Geometry: final body of the model. Coordinates: model frame, mm. A direction names the side the tool comes from. Give positions to 0.01 mm unless a question says otherwise; leave off trailing zeros. Loops run counter-clockwise (first coordinate to the right, second up) from the corner with the lowest first, then second, coordinate; pieces in that order, holes last. Notation, with made-up numbers: M 76,-18 L 126,-18 A18 cw 126,11 Z; hole C 83,-23.75 d8. An arc over 180 degrees is marked long. Put each result on its own line as item: value.
```python
from build123d import *

# Parameters (mm, degrees)
SKETCH2_W                = 10
SKETCH2_H                = 7.3
BOSS_EXTRUDE1_DEPTH      = 4.55
SKETCH3_W                = 4.6
SKETCH3_H                = 4.9
CUT_EXTRUDE1_DEPTH       = 3.3
BOSS_EXTRUDE2_DEPTH      = 9.55
BOSS_EXTRUDE2_DEPTH_BACK = 2.7
SKETCH5_W                = 4
SKETCH5_H                = 2
BOSS_EXTRUDE3_REACH      = 19.417
SKETCH13_W               = 5
SKETCH13_H               = 2
SKETCH6_W                = 1.74
SKETCH6_H                = 2
SKETCH6_W_2              = 0.86
SKETCH6_W_3              = 0.8
BOSS_EXTRUDE4_DEPTH      = 0.8
FILLET1_R                = 5
CUT_EXTRUDE2_DEPTH       = 1.2
SKETCH8_R                = 0.65
CUT_EXTRUDE3_DEPTH       = 15.703826033
SKETCH9_R                = 1.125
CUT_EXTRUDE4_DEPTH       = 15.670122699
CUT_EXTRUDE5_REACH       = 20.001
SKETCH10_R               = 0.65
CUT_EXTRUDE6_DEPTH       = 1.3
SKETCH14_W               = 3.4
SKETCH14_H               = 2.947905619
BOSS_EXTRUDE6_DEPTH      = 1.5
SKETCH15_W               = 1.5
SKETCH15_H               = 1.602094381
CUT_EXTRUDE7_DEPTH       = 1.5
FILLET2_R                = 0.25
SKETCH16_W               = 5.8
SKETCH16_H               = 4.9
CUT_EXTRUDE8_DEPTH       = 0.7


with BuildPart() as part:
    # Sketch2 → Boss-Extrude1 (new body)
    with BuildSketch(Plane.XY):
        with Locations((5, 3.65)):
            Rectangle(SKETCH2_W, SKETCH2_H)
    extrude(amount=BOSS_EXTRUDE1_DEPTH)

    # Sketch3 → Cut-Extrude1 (cut)
    with BuildSketch(Plane.XY.offset(4.55)):
        with Locations((4.3, 2.45)):
            Rectangle(SKETCH3_W, SKETCH3_H)
    extrude(amount=-CUT_EXTRUDE1_DEPTH, mode=Mode.SUBTRACT)

    # Sketch5 → Boss-Extrude2 (add, two sides: drawn at the far end of the back side and taken through both)
    with BuildSketch(Plane.XY.offset(-BOSS_EXTRUDE2_DEPTH_BACK)):
        with Locations((-1.4, 4.8)):
            Rectangle(SKETCH5_W, SKETCH5_H)
    extrude(amount=BOSS_EXTRUDE2_DEPTH + BOSS_EXTRUDE2_DEPTH_BACK)

    # Sketch13 → Boss-Extrude3 (add, up to next)
    with BuildSketch(Plane(origin=(0, 0, -2.7), x_dir=(-1, 0, 0), z_dir=(0, 0, -1)), mode=Mode.PRIVATE) as boss_extrude3_sk1:
        with Locations((0.9, 4.8)):
            Rectangle(SKETCH13_W, SKETCH13_H)
    boss_extrude3_tool1 = extrude(boss_extrude3_sk1.sketch, amount=-BOSS_EXTRUDE3_REACH, mode=Mode.PRIVATE) - part.part
    add(boss_extrude3_tool1.solids().sort_by_distance((-0.9, 4.8, -2.7))[0])

    # Sketch6 → Boss-Extrude4 (add)
    with BuildSketch(Plane(origin=(0, 0, -2.7), x_dir=(-1, 0, 0), z_dir=(0, 0, -1))):
        with Locations((0.93, 4.8)):
            Rectangle(SKETCH6_W, SKETCH6_H)
        with Locations((-1.17, 4.8)):
            Rectangle(SKETCH6_W_2, SKETCH6_H)
        with Locations((3, 4.8)):
            Rectangle(SKETCH6_W_3, SKETCH6_H)
    extrude(amount=BOSS_EXTRUDE4_DEPTH)

    # Fillet1
    # the kernel refuses this fillet: 5 mm, written as the material it adds along each edge
    with BuildSketch(Plane(origin=(1.6, 3.8, 0), x_dir=(0, 0, -1), z_dir=(0, 1, 0))) as fillet1_piece_1:
        with BuildLine():
            CenterArc((5, -4.769696007), FILLET1_R, 107.457603124, 72.542396876)
            Line((0, -4.769696007), (-0.1, -4.769696007))
            Line((-0.1, -4.769696007), (-0.1, 0))
            Line((-0.1, 0), (0, 0.1))
            ThreePointArc((0, 0.1), (1.75, 0.1), (3.47, 0.09539392))
            Line((3.47, 0.09539392), (3.5, 0))
        make_face()
    extrude(amount=2)

    # Sketch7 → Cut-Extrude2 (cut)
    with BuildSketch(Plane(origin=(0, 3.8, 0), x_dir=(-1, 0, 0), z_dir=(0, -1, 0))):
        Polygon((0.25, -7.138141571), (0.25, -8.46604719), (1.4, -9.13), (2.55, -8.46604719), (2.55, -7.138141571), (1.4, -6.474188762), align=None)
        Polygon((1.4, 1.125811238), (0.25, 0.461858429), (0.25, -0.86604719), (1.4, -1.53), (2.55, -0.86604719), (2.55, 0.461858429), align=None)
    extrude(amount=-CUT_EXTRUDE2_DEPTH, mode=Mode.SUBTRACT)

    # Sketch8 → Cut-Extrude3 (cut, through all)
    with BuildSketch(Plane.XZ.offset(-5)):
        with Locations(Location((-1.4, 7.802094381, 0), (0, 0, 270))):
            Circle(SKETCH8_R)
        with Locations(Location((-1.4, 0.202094381, 0), (0, 0, 270))):
            Circle(SKETCH8_R)
    extrude(amount=-CUT_EXTRUDE3_DEPTH, mode=Mode.SUBTRACT)

    # Sketch9 → Cut-Extrude4 (cut, through all)
    with BuildSketch(Plane.XZ.offset(-4.9)):
        with Locations(Location((3.5, 2.75, 0), (0, 0, 270))):
            Circle(SKETCH9_R)
    extrude(amount=-CUT_EXTRUDE4_DEPTH, mode=Mode.SUBTRACT)

    # Sketch10 → Cut-Extrude5 (cut, up to next)
    with BuildSketch(Plane(origin=(10, 0, 0), x_dir=(0, 0, -1), z_dir=(1, 0, 0)), mode=Mode.PRIVATE) as cut_extrude5_sk1:
        with Locations((-2.625, 3.5)):
            Circle(SKETCH10_R)
    cut_extrude5_tool1 = extrude(cut_extrude5_sk1.sketch, amount=-CUT_EXTRUDE5_REACH, mode=Mode.PRIVATE) & part.part
    add(cut_extrude5_tool1.solids().sort_by_distance((10, 3.5, 2.625))[0], mode=Mode.SUBTRACT)

    # Sketch12 → Cut-Extrude6 (cut)
    with BuildSketch(Plane(origin=(9, 0, 0), x_dir=(0, 0, -1), z_dir=(1, 0, 0))):
        Polygon((-3.257198545, 2.405), (-4.55, 2.405), (-4.55, 4.595), (-3.257198545, 4.595), (-1.992801455, 4.595), (-1.36060291, 3.5), (-1.992801455, 2.405), align=None)
    extrude(amount=-CUT_EXTRUDE6_DEPTH, mode=Mode.SUBTRACT)

    # Sketch14 → Boss-Extrude6 (add)
    with BuildSketch(Plane(origin=(0, 5.8, 0), x_dir=(1, 0, 0), z_dir=(0, 1, 0))):
        with Locations((-1.7, -3.076047191)):
            Rectangle(SKETCH14_W, SKETCH14_H)
    extrude(amount=BOSS_EXTRUDE6_DEPTH)

    # Sketch15 → Cut-Extrude7 (cut)
    with BuildSketch(Plane(origin=(0, 7.3, 0), x_dir=(1, 0, 0), z_dir=(0, 1, 0))):
        with Locations((0.75, -0.801047191)):
            Rectangle(SKETCH15_W, SKETCH15_H)
    extrude(amount=-CUT_EXTRUDE7_DEPTH, mode=Mode.SUBTRACT)

    # Fillet2
    fillet2_edges = [part.edges().sort_by_distance(p)[0] for p in [
        (3.3, 7.3, 4.55),
        (-0.95, 7.3, 1.602094381),
    ]]
    fillet(fillet2_edges, radius=FILLET2_R)

    # Sketch16 → Cut-Extrude8 (cut)
    with BuildSketch(Plane.XY.offset(4.55)):
        with Locations((4.3, 2.45)):
            Rectangle(SKETCH16_W, SKETCH16_H)
    extrude(amount=-CUT_EXTRUDE8_DEPTH, mode=Mode.SUBTRACT)


solid = part.part
```
Item 1: Mould query, pull axis Z, two halves, no side actions, for faces 1 (the flat face through (-1, 5, -3.5)), 2 (the flat face through (-0.817, 4.392, 1.193)), 3 (the flat face through (10, 4, 2)). Classes: pulls with the +Z half, pulls with the -Z half, needs draft (parallel to the pull), parting line crosses it, or undercut.
Output values:
face 1: pulls with the -Z half
face 2: undercut
face 3: needs draft
Item 2: Section D-D on z = 2.75. Output: boundary loops of the cut face in (x, y) (3 decimals).
Output values:
outline: M -3.4,3.8 L 0,3.8 L 0,0 L 2,0 L 2,4.9 L 2.375,4.9 L 2.375,7.3 L -3.4,7.3 Z; M 4.625,4.9 L 6.6,4.9 L 6.6,4.138 L 7.7,4.138 L 7.7,4.595 L 9,4.595 L 9,4.138 L 10,4.138 L 10,7.3 L 4.625,7.3 Z; M 6.6,0 L 10,0 L 10,2.862 L 9,2.862 L 9,2.405 L 7.7,2.405 L 7.7,2.862 L 6.6,2.862 Z
Item 3: Pin query (flat end, axial travel): pin 1 Ø1.7 at (x, z) = (-1.4, 0.2) entering from +Y; pin 2 Ø3 at (y, z) = (1, 2) entering from -X; pin 3 Ø1.2 at (x, z) = (-1, 1) entering from -Y. Return the tip coordinate at first contact, or that it passes through.
Output values:
pin 1: y = 5.8
pin 2: x = 0
pin 3: y = 3.8
Item 4: Set-up query: faces 4 (the cylindrical face through (9.51, 2.92, 2.33)), 5 (the flat face through (1.5, 7, 1)), 6 (the flat face through (8.359, 2.96, 1.672)), 7 (the flat face through (-1.97, 4.39, 8.8)). Return all of +Z, -Z, +X, -X, +Y, -Y with unobstructed straight access to the full face (end or side cutting, diameter ignored); none if empty.
Output values:
face 4: +X
face 5: -Z, -X, +Y
face 6: +Z
face 7: -Y
Item 5: Section B-B on y = 0.75. Output: boundary loops of the cut face in (x, z).
Output values:
outline: M 0,0 L 10,0 L 10,4.55 L 7.2,4.55 L 7.2,3.85 L 6.6,3.85 L 6.6,1.25 L 2,1.25 L 2,3.85 L 1.4,3.85 L 1.4,4.55 L 0,4.55 Z
Item 6: Line query: probe 1 along X at (y, z) = (3.5, 1.75); probe 2 along Z at (x, y) = (3.5, 6.5) (3 decimals); probe 3 along Y at (x, z) = (-1.75, 2). Output: solid intervals per line, ascending. Write a range as [from, to].
Output values:
probe 1: [0, 2], [6.6, 7.7], [9, 10]
probe 2: [0, 1.625], [3.875, 4.55]
probe 3: [3.8, 7.3]
Item 7: Section C-C on x = 3. Output: boundary loops of the cut face in (y, z), then the cut area to 3 significant figures.
Output values:
outline: M 0,0 L 3.8,0 L 3.8,-1.31 L 5.8,-1.31 L 5.8,0 L 7.3,0 L 7.3,1.74 L 4.9,1.74 L 4.9,1.25 L 0,1.25 Z; M 4.9,3.76 L 7.3,3.76 L 7.3,4.3 A0.25 ccw 7.05,4.55 L 4.9,4.55 Z
area: 14.8 mm²
Item 8: Section A-A on y = 5.5. Output: boundary loops of the cut face in (x, z) (3 decimals), then the cut area to 3 significant figures.
Output values:
outline: M -3.4,-3.5 L -2.6,-3.5 L -2.6,-2.7 L -1.8,-2.7 L -1.8,-3.5 L -0.06,-3.5 L -0.06,-2.7 L 0.74,-2.7 L 0.74,-3.5 L 1.6,-3.5 A5 cw 6.37,0 L 10,0 L 10,4.55 L 0.6,4.55 L 0.6,9.55 L -3.4,9.55 Z; hole C -1.4,0.202 d1.3; hole C -1.4,7.802 d1.3; hole C 3.5,2.75 d2.25
area: 95.0 mm²
